Autodesk Inventor part; units mm, degrees
ref_plane "YZ Plane" through (0, 0, 0) normal (1, 0, 0) x (0, 1, 0)
ref_plane "XZ Plane" through (0, 0, 0) normal (0, 1, 0) x (-1, 0, 0)
ref_plane "XY Plane" through (0, 0, 0) normal (0, 0, 1) x (1, 0, 0)
sketch "スケッチ1" plane through (0, 0, 0) normal (0, 0, 1) x (1, 0, 0)
  line L0 (0, 0) -> (30, 0)
  line L1 (30, 0) -> (30, 94)
  line L2 (30, 94) -> (0, 94)
  line L3 (0, 94) -> (0, 0)
  dimension "d0" = 30
  dimension "d1" = 94
extrude "プレート1" add sketch "スケッチ1" along normal blind 1.5
sketch "スケッチ2" plane through (0, 0, 1.5) normal (0, 0, 1) x (1, 0, 0)
  line L0 (30, 94) -> (30, 0)
  circle A0 centre (10, 47) radius 1.6
  circle A1 centre (20, 47) radius 1.6
  line L1 (30, 0) -> (0, 0)
  line L2 (30, 94) -> (30, 0)
  line L3 (0, 94) -> (30, 94)
  line L4 (0, 0) -> (0, 94)
  line L5 (15, 94) -> (15, 0)
  circle A2 centre (20, 17) radius 1.6
  circle A3 centre (10, 17) radius 1.6
  circle A4 centre (20, 77) radius 1.6
  circle A5 centre (10, 77) radius 1.6
  circle A6 centre (20, 47) radius 1.6
  circle A7 centre (10, 47) radius 1.6
  point P0 (30, 47)
  dimension "d3" = 3.2
  dimension "d4" = 3.2
  dimension "d5" = 10
  dimension "d8" = 30
  dimension "d11" = 30
extrude "切り取り1" cut sketch "スケッチ2" against normal blind 1.5 contours A0 | A1 | A2 | A3 | A4 | A5
equation "\"d14\" = Thickness"
equation "\"d2\" = Thickness"
equation "\"BendRadius\" = Thickness"
equation "\"BendReliefWidth\" = Thickness"
equation "\"BendReliefDepth\" = 0.5 * Thickness"
equation "\"CornerReliefSize\" = 4 * Thickness"
equation "\"MinimumRemnant\" = 2 * Thickness"
equation "\"TransitionRadius\" = BendRadius"
equation "\"JacobiRadiusSize\" = BendRadius"
equation "\"GapSize\" = Thickness"
properties part number "rail_rail" material "アルミニウム 6061"
Here's how the part is built. I have some questions about the finished solid (model axes, mm). Round coordinates to 2 decimals unless told otherwise and drop trailing zeros. Loops run counter-clockwise (first coordinate to the right, second up) from the corner with the lowest first, then second, coordinate; pieces in that order, holes last. Notation, with made-up numbers: M -32.75,9 L -8.75,9 A17 cw -8.75,15 Z; hole C 54.5,62.25 d11. An arc over 180 degrees is marked long. Write each question's results on one line, items separated by ' | '. Start each with the question number.
(1) I want a section at D-D (x = 20.25). Please give me the cut outline in (y, z), then the cut area to 3 significant figures.
(2) If I drill on probe 1 along Y at (x, z) = (10, 0.9); probe 2 along X at (y, z) = (77, 1.1); probe 3 along X at (y, z) = (18, 0.4), over which ranges is the centre line in solid material (lowest first)? Write a range as from..to.
(3) I want a section at B-B (z = 1.25). Please give me the cut outline in (x, y), then the cut area to 3 significant figures.
(4) I want a section at C-C (y = 47). Please give me the cut outline in (x, z), then the cut area to 3 significant figures.
(5) I want a section at A-A (x = 10). Please give me the cut outline in (y, z).
(6) Thinking about a two-plate mould opening in Y: for faces 1 (the flat face through (30, 46, 1)), 2 (the flat face through (15, 0, 1)), 3 (the cylindrical face through (19.792, 18.586, 0.76)), which applies, pulls with the +Y half, pulls with the -Y half, needs draft (parallel to the pull), parting line crosses it, or undercut?
(7) Will this pin go through, and if not, where does the flat tip stop? P1, Ø2.5, axis at x = 10, y = 77, coming from the -Z side.
Solved:
1) outline: M 0,0 L 15.42,0 L 15.42,1.5 L 0,1.5 Z; M 18.58,0 L 45.42,0 L 45.42,1.5 L 18.58,1.5 Z; M 48.58,0 L 75.42,0 L 75.42,1.5 L 48.58,1.5 Z; M 78.58,0 L 94,0 L 94,1.5 L 78.58,1.5 Z | area: 127 mm²
2) probe 1: y = 0..15.4, 18.6..45.4, 48.6..75.4, 78.6..94 | probe 2: x = 0..8.4, 11.6..18.4, 21.6..30 | probe 3: x = 0..8.75, 11.25..18.75, 21.25..30
3) outline: M 0,0 L 30,0 L 30,94 L 0,94 Z; hole C 10,17 d3.2; hole C 10,47 d3.2; hole C 10,77 d3.2; hole C 20,17 d3.2; hole C 20,47 d3.2; hole C 20,77 d3.2 | area: 2,770 mm²
4) outline: M 0,0 L 8.4,0 L 8.4,1.5 L 0,1.5 Z; M 11.6,0 L 18.4,0 L 18.4,1.5 L 11.6,1.5 Z; M 21.6,0 L 30,0 L 30,1.5 L 21.6,1.5 Z | area: 35.4 mm²
5) outline: M 0,0 L 15.4,0 L 15.4,1.5 L 0,1.5 Z; M 18.6,0 L 45.4,0 L 45.4,1.5 L 18.6,1.5 Z; M 48.6,0 L 75.4,0 L 75.4,1.5 L 48.6,1.5 Z; M 78.6,0 L 94,0 L 94,1.5 L 78.6,1.5 Z
6) face 1: needs draft | face 2: pulls with the -Y half | face 3: undercut
7) P1: passes through
